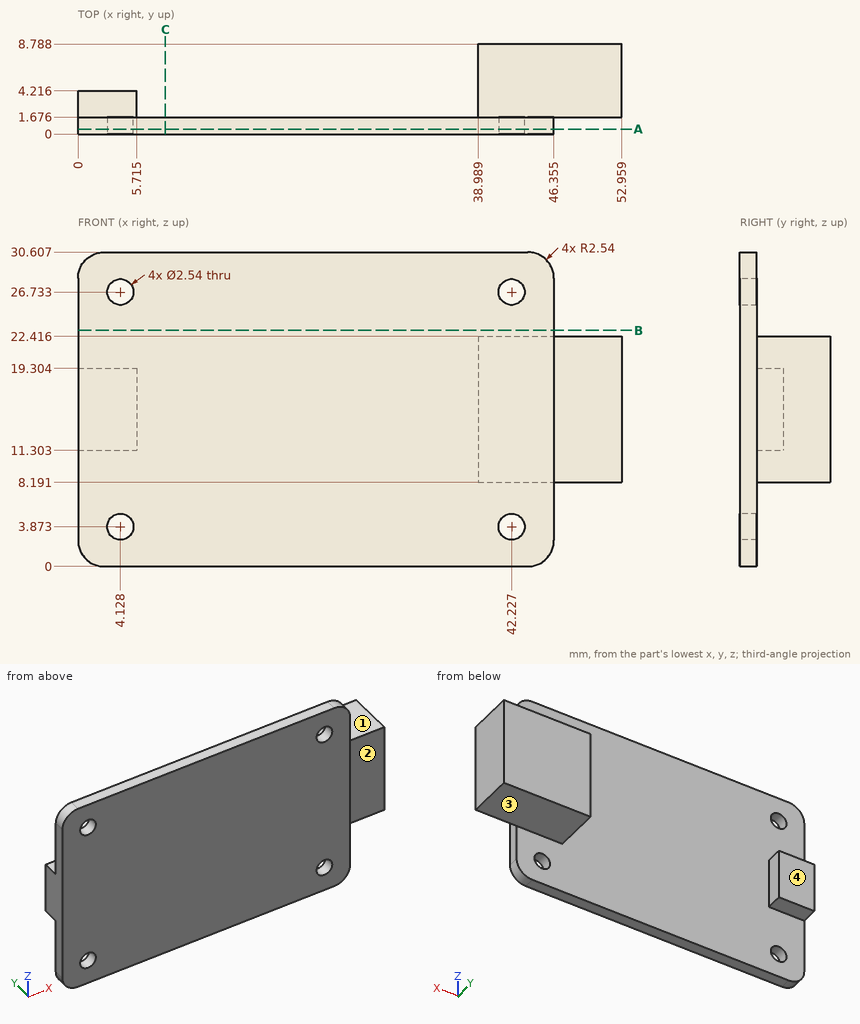
The figure shows three views and two pictorial views of one solid part (mm, origin at its lowest corner). Answer the questions. A direction names the side the tool comes from. Round coordinates to 2 decimals unless told otherwise and drop trailing zeros. Write each loop counter-clockwise with the first axis right and the second up, starting at its lowest first coordinate (ties: lowest second). Pieces come first, ordered by that corner, then holes. Notation, with made-up numbers: M 61,-39 L 71,-39 A3 ccw 71,-34 Z; hole C 61.5,-24.75 d3. An arc over 180 degrees is marked long. Write each question's results on one line, items separated by ' | '. Start each with the question number.
(1) Each of these flat-tipped pins is pushed along its axis until it touches: P1, Ø2, axis at x = 43, y = 6, coming from the -Z side; P2, Ø1.5, axis at y = 5, z = 17, coming from the -X side; P3, Ø2, axis at x = 45.5, y = 4, coming from the +Z side (1 decimal). Where does it stop, or does it pass through?
(2) Find the intervals of material crossed by line 1 (X direction, y = 1, z = 4) (1 decimal); line 2 (Z direction, x = 42, y = 0.5) (1 decimal); line 3 (Y direction, x = 33, z = 11.5), in increasing order.
(3) The part is cut by section C-C, the plane x = 8.5. Write down the section's boundary in (y, z).
(4) The part is cut by section A-A, the plane y = 0.5. Write down the section's boundary in (x, z) (1 decimal), and give its area (3 significant figures).
(5) For the marked faces 1, 2, 3 and 4, determine the directions among +Z, -Z, +X, -X, +Y, -Y from which every point of the face is accessible in a straight line to the end or side of a thin tool.
(6) The part is cut by section B-B, the plane z = 23. Write down the section's boundary in (x, y) (1 decimal).
Worked answers:
1) P1: stops at z = 8.19 | P2: stops at x = 38.99 | P3: stops at z = 22.4
2) line 1: x = 0 to 2.9, 5.4 to 41, 43.5 to 46.4 | line 2: z = 0 to 2.6, 5.1 to 25.5, 28 to 30.6 | line 3: y = 0 to 1.68
3) outline: M 0,0 L 1.68,0 L 1.68,30.61 L 0,30.61 Z
4) outline: M 0,2.5 A2.5 ccw 2.5,0 L 43.8,0 A2.5 ccw 46.4,2.5 L 46.4,28.1 A2.5 ccw 43.8,30.6 L 2.5,30.6 A2.5 ccw 0,28.1 Z; hole C 4.1,3.9 d2.5; hole C 4.1,26.7 d2.5; hole C 42.2,3.9 d2.5; hole C 42.2,26.7 d2.5 | area: 1,390 mm²
5) face 1: +Z, +X, -X, +Y | face 2: +Z, -Z, +X, -Y | face 3: -Z, +X, -X, +Y | face 4: +Z, -Z, -X, +Y
6) outline: M 0,0 L 46.4,0 L 46.4,1.7 L 0,1.7 Z
